```python
from build123d import *

# Parameters (mm, degrees)
F0_R     = 10
F1_DEPTH = 25
F2_DEPTH = 50
F3_SIZE  = 2
F4_W     = 54.479554
F4_H     = 43.313496
F5_DEPTH = 25


with BuildPart() as f1:
    # F0 (on Front) → F1 (new body)
    with BuildSketch(Plane.XZ):
        with BuildLine():
            ThreePointArc((2.083333, -24.913043), (18.399502, -16.92508), (25, 0))
            ThreePointArc((25, 0), (18.399502, 16.92508), (2.083333, 24.913043))
            ThreePointArc((2.083333, 24.913043), (-25, 0), (2.083333, -24.913043))
        make_face()
        Circle(F0_R, mode=Mode.SUBTRACT)
        with BuildLine():
            ThreePointArc((2.083333, 24.913043), (18.399502, 16.92508), (25, 0))
            ThreePointArc((25, 0), (18.399502, -16.92508), (2.083333, -24.913043))
            Line((2.083333, -24.913043), (91.458333, -17.43913))
            ThreePointArc((91.458333, -17.43913), (72.5, 0), (91.458333, 17.43913))
            Line((91.458333, 17.43913), (2.083333, 24.913043))
        make_face()
        with BuildLine():
            ThreePointArc((107.5, 0), (102.879651, 11.847556), (91.458333, 17.43913))
            ThreePointArc((91.458333, 17.43913), (72.5, 0), (91.458333, -17.43913))
            ThreePointArc((91.458333, -17.43913), (102.879651, -11.847556), (107.5, 0))
        make_face()
        with Locations((90, 0)):
            Circle(F0_R, mode=Mode.SUBTRACT)
    extrude(amount=F1_DEPTH)

    # F0 (on Front) → F2 (join)
    with BuildSketch(Plane.XZ):
        with BuildLine():
            ThreePointArc((2.083333, -24.913043), (18.399502, -16.92508), (25, 0))
            ThreePointArc((25, 0), (18.399502, 16.92508), (2.083333, 24.913043))
            ThreePointArc((2.083333, 24.913043), (-25, 0), (2.083333, -24.913043))
        make_face()
        Circle(F0_R, mode=Mode.SUBTRACT)
    extrude(amount=F2_DEPTH)

    # F3
    f3_edges = [f1.edges().sort_by_distance(p)[0] for p in [
        (-2.083333, -50, 24.913043),
        (-10, -50, 0),
        (80, -25, 0),
    ]]
    chamfer(f3_edges, length=F3_SIZE)

    # F4 (on Top) → F5 (join)
    with BuildSketch(Plane.XY):
        with Locations((27.239777, 21.656748)):
            Rectangle(F4_W, F4_H)
    extrude(amount=F5_DEPTH)


solid = f1.part
```
Input: part model. Units: mm. Frame: model coordinates. A direction names the side the tool comes from. Round coordinates to 2 decimals unless told otherwise and drop trailing zeros. Loops run counter-clockwise (first coordinate to the right, second up) from the corner with the lowest first, then second, coordinate; pieces in that order, holes last. Notation, with made-up numbers: (39, 63.5) -> (77, 63.5) arc R31 cw to (77, 98.5) -> close; hole circle Ø2 at (-11, 30). An arc over 180 degrees is marked (long way). Use one line per item in the form item = value. Start each with the question number.
Item 1: Mould query, pull axis X, two halves, no side actions, for faces 5 (the face through (10, -50, -10)), 6 (the face through (47.396, -12.325, 21.124)), 7 (the face through (81.965, -23.125, -6.161)), 8 (the face through (-2.17, -23.66, -9.76)). Classes: pulls with the +X half, pulls with the -X half, needs draft (parallel to the pull), parting line crosses it, or undercut.
Item 2: Set-up query: faces 1 (the face through (39, 0, 24)), 2 (the face through (0, 21, 12)), 3 (the face through (54.48, 21, 12)), 4 (the face through (4, 0, 4)). Return all of +Z, -Z, +X, -X, +Y, -Y with unobstructed straight access to the full face (end or side cutting, diameter ignored); none if empty.
Item 3: Contact query for flat-ended pins moving along their axis: pin 1 Ø8 at (x, z) = (87, -14.5) entering from +Y; pin 2 Ø8 at (x, z) = (4.5, 4.5) entering from -Y; pin 3 Ø3.5 at (x, z) = (22.5, 22.5) entering from -Y. Output: stop coordinate, or through.
Item 4: Section query B-B on y = -15. Return the cut outline in (x, z), then the cut area to 3 significant figures.
Item 5: Section query D-D on y = -27. Return the cut outline in (x, z), then the cut area to 3 significant figures.
Item 6: Section query C-C on x = 40. Return the cut outline in (y, z).
Item 7: Material intervals for L1, parallel to Z at x = 0, y = -32; L2, parallel to Z at x = 23.5, y = 38, sorted ascending. Write a range as from..to.
Item 8: Section query A-A on x = 90. Return the cut outline in (y, z), then the cut area to 3 significant figures.
Ans:
q1.face_5 = needs draft
q1.face_6 = pulls with the +X half
q1.face_7 = undercut
q1.face_8 = undercut
q2.face_1 = +Z, +X, -Y
q2.face_2 = +Z, -Z, -X, +Y
q2.face_3 = +Z, -Z, +X, +Y
q2.face_4 = -Y
q3.pin_1 = 0
q3.pin_2 = -48.36
q3.pin_3 = -25
q4.outline = (2.08, -24.91) -> (91.46, -17.44) arc R17.5 ccw to (91.46, 17.44) -> (2.08, 24.91) arc R25 ccw (long way) to start; hole circle Ø20 at (0, 0); hole circle Ø20 at (90, 0)
q4.area = 4,670 mm^2
q5.outline = (2.08, -24.91) arc R25 ccw to (25, 0) arc R25 ccw to (2.08, 24.91) arc R25 ccw (long way) to start; hole circle Ø20 at (0, 0)
q5.area = 1,650 mm^2
q6.outline = (-25, -21.74) -> (0, -21.74) -> (0, 0) -> (43.31, 0) -> (43.31, 25) -> (0, 25) -> (0, 21.74) -> (-25, 21.74) -> close
q7.L1 = -25..-10, 10..25
q7.L2 = 0..25
q8.outline = (-25, -17.56) -> (0, -17.56) -> (0, -10) -> (-23, -10) -> (-25, -12) -> close; (-25, 12) -> (-23, 10) -> (0, 10) -> (0, 17.56) -> (-25, 17.56) -> close
q8.area = 374 mm^2
